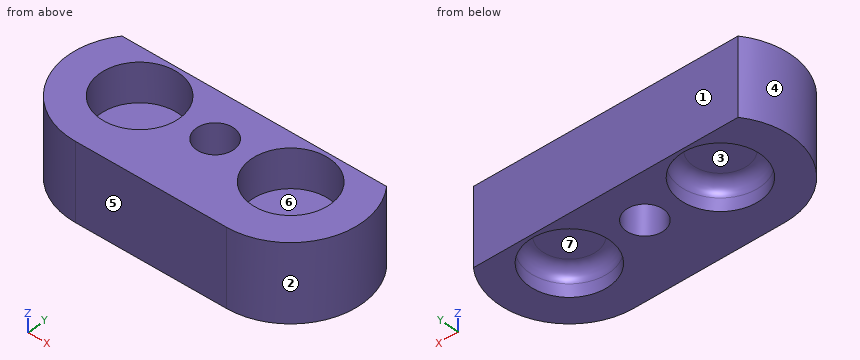
from build123d import *

# Parameters (mm, degrees)
SKETCH1_R           = 3.5
SKETCH1_R_2         = 3.1
EXTRUDE_THIN1_DEPTH = 2
BOSS_EXTRUDE1_DEPTH = 4
SKETCH3_R           = 3.05
CUT_EXTRUDE1_DEPTH  = 3
CUT_EXTRUDE2_REACH  = 15.016
SKETCH4_R           = 1.45
BOSS_EXTRUDE2_START = 2
SKETCH5_R           = 1.45
BOSS_EXTRUDE2_DEPTH = 2
FILLET1_R           = 1
EXTRUDE_THIN2_START = -6
EXTRUDE_THIN2_DEPTH = 6
CUT_EXTRUDE3_REACH  = 17.557


with BuildPart() as part:
    # Sketch1 → Extrude-Thin1 (new body)
    with BuildSketch(Plane.XY):
        with Locations((-5.8, 3.35)):
            Circle(SKETCH1_R)
        with Locations((-5.8, 3.35)):
            Circle(SKETCH1_R_2, mode=Mode.SUBTRACT)
    extrude(amount=EXTRUDE_THIN1_DEPTH)


with BuildPart() as body_2:
    # Mirror3: mirrored copy
    add(part.part.mirror(Plane(origin=(0, 0, 0), x_dir=(0, 0, 1), z_dir=(1, 0, 0))))


with BuildPart() as part_1:
    add(part.part)

    add(body_2.part)  # Boss-Extrude1 merges body 2
    # Sketch2 → Boss-Extrude1 (add)
    with BuildSketch(Plane.XY.offset(2)):
        with BuildLine():
            Line((-5.8, 6.85), (5.8, 6.85))
            ThreePointArc((5.8, 6.85), (9.3, 3.35), (5.8, -0.15))
            Line((5.8, -0.15), (-5.8, -0.15))
            ThreePointArc((-5.8, -0.15), (-9.3, 3.35), (-5.8, 6.85))
        make_face()
    extrude(amount=BOSS_EXTRUDE1_DEPTH)

    # Sketch3 → Cut-Extrude1 (cut)
    with BuildSketch(Plane.XY.offset(6)):
        with Locations((-5.8, 3.35)):
            Circle(SKETCH3_R)
    cut_extrude1 = extrude(amount=-CUT_EXTRUDE1_DEPTH, mode=Mode.SUBTRACT)

    # Mirror4: Cut-Extrude1 across plane
    add(cut_extrude1.mirror(Plane(origin=(0, 0, 0), x_dir=(0, 0, 1), z_dir=(1, 0, 0))), mode=Mode.SUBTRACT)

    # Sketch4 → Cut-Extrude2 (cut, up to next)
    with BuildSketch(Plane.XY.offset(6), mode=Mode.PRIVATE) as cut_extrude2_sk1:
        with Locations((0, 3.35)):
            Circle(SKETCH4_R)
    cut_extrude2_tool1 = extrude(cut_extrude2_sk1.sketch, amount=-CUT_EXTRUDE2_REACH, mode=Mode.PRIVATE) & part_1.part
    add(cut_extrude2_tool1.solids().sort_by_distance((0, 3.35, 6))[0], mode=Mode.SUBTRACT)

    # Sketch5 → Boss-Extrude2 (add)
    with BuildSketch(Plane(origin=(0, 0, 2), x_dir=(-1, 0, 0), z_dir=(0, 0, -1)).offset(BOSS_EXTRUDE2_START)):
        with BuildLine():
            Line((-5.8, -0.15), (5.8, -0.15))
            ThreePointArc((5.8, -0.15), (2.3, 3.35), (5.8, 6.85))
            Line((5.8, 6.85), (-5.8, 6.85))
            ThreePointArc((-5.8, 6.85), (-2.3, 3.35), (-5.8, -0.15))
        make_face()
        with Locations(Location((0, 3.35, 0), (0, 0, 180))):
            Circle(SKETCH5_R, mode=Mode.SUBTRACT)
    extrude(amount=-BOSS_EXTRUDE2_DEPTH)

    # Fillet1
    fillet1_edges = [part_1.edges().sort_by_distance(p)[0] for p in [
        (-8.9, 3.35, 2),
        (8.9, 3.35, 2),
    ]]
    fillet(fillet1_edges, radius=FILLET1_R)

    # Sketch6 → Extrude-Thin2 (add)
    with BuildSketch(Plane.XY.offset(6).offset(EXTRUDE_THIN2_START)):
        with BuildLine():
            Line((5.8, 8.85), (-5.8, 8.85))
            ThreePointArc((-5.8, 8.85), (-11.3, 3.35), (-5.8, -2.15))
            Line((-5.8, -2.15), (5.8, -2.15))
            ThreePointArc((5.8, -2.15), (11.3, 3.35), (5.8, 8.85))
        make_face()
        with BuildLine():
            Line((5.8, 6.85), (-5.8, 6.85))
            ThreePointArc((-5.8, 6.85), (-9.3, 3.35), (-5.8, -0.15))
            Line((-5.8, -0.15), (5.8, -0.15))
            ThreePointArc((5.8, -0.15), (9.3, 3.35), (5.8, 6.85))
        make_face(mode=Mode.SUBTRACT)
    extrude(amount=EXTRUDE_THIN2_DEPTH)

    # Sketch7 → Cut-Extrude3 (cut, up to next)
    with BuildSketch(Plane.XY.offset(6), mode=Mode.PRIVATE) as cut_extrude3_sk1:
        with BuildLine():
            Line((-10.162052269, 6.7), (10.162052269, 6.7))
            ThreePointArc((10.162052269, 6.7), (8.231563283, 8.28330518), (5.8, 8.85))
            Line((5.8, 8.85), (-5.8, 8.85))
            ThreePointArc((-5.8, 8.85), (-8.231563283, 8.28330518), (-10.162052269, 6.7))
        make_face()
    cut_extrude3_tool1 = extrude(cut_extrude3_sk1.sketch, amount=-CUT_EXTRUDE3_REACH, mode=Mode.PRIVATE) & part_1.part
    add(cut_extrude3_tool1.solids().sort_by_distance((0, 7.706585, 6))[0], mode=Mode.SUBTRACT)


solid = part_1.part
Geometry: final body of the model. Coordinates: model frame, mm. Face numbers are marked on the shaded views. A direction names the side the tool comes from. Round coordinates to 2 decimals unless told otherwise and drop trailing zeros. Order: outer loops, then holes, each group sorted by start corner. A loop starts at its lowest first (then second) coordinate and runs counter-clockwise, first axis right, second up. Notation, with made-up numbers: (-32, 49.25) -> (23, 49.25) arc R32 ccw to (23, 87.25) -> close; hole circle Ø9 at (-38.75, 76). An arc over 180 degrees is marked (long way). Put each result on its own line as item: value. Start each with the question number.
Q1. Section C-C on z = 4.75. Return the cut outline in (x, y).
Q2. Section A-A on y = 3.35. Return the cut outline in (x, z), and give its area (3 significant figures).
Q3. Reachability of the marked faces 5, 6 and 7 from +Z, -Z, +X, -X, +Y, -Y: full face, straight path, thin tool, end or side. Return the list, or none.
Q4. Section D-D on z = 0.5. Return the cut outline in (x, y), and give its area (3 significant figures).
Q5. First-contact query: pin 1 (2 mm diameter, centred on y = 2, z = 1, fed in from -X); pin 2 (5 mm diameter, centred on x = 7.5, y = 3.5, fed in from +Z); pin 3 (5 mm diameter, centred on x = -5.8, y = 3.35, fed in from +Z); pin 4 (4.5 mm diameter, centred on x = -5.5, y = 3.5, fed in from -Z). Flat tips, straight axial feed; report the tip coordinate or a pass-through.
Q6. Line query: probe 1 along X at (y, z) = (3.35, 2.7); probe 2 along Y at (x, z) = (5.8, 3.95); probe 3 along X at (y, z) = (5, 0.8). Output: solid intervals per line, ascending.
Q7. Pull-direction query (X, two-part tool) for the marked faces 1, 2, 3 and 4; classes: +X half, -X half, draft (parallel to the pull), parting line (faces both ways), or undercut.
Q8. Section B-B on x = 0. Return the cut outline in (y, z).
Ans:
1. outline: (-10.16, 6.7) arc R5.5 ccw to (-5.8, -2.15) -> (5.8, -2.15) arc R5.5 ccw to (10.16, 6.7) -> close; hole circle Ø6.1 at (-5.8, 3.35); hole circle Ø2.9 at (0, 3.35); hole circle Ø6.1 at (5.8, 3.35)
2. outline: (-11.3, 0) -> (-8.9, 0) -> (-8.9, 1) arc R1 cw to (-7.9, 2) -> (-3.7, 2) arc R1 cw to (-2.7, 1) -> (-2.7, 0) -> (-1.45, 0) -> (-1.45, 6) -> (-2.75, 6) -> (-2.75, 3) -> (-8.85, 3) -> (-8.85, 6) -> (-11.3, 6) -> close; (1.45, 0) -> (2.7, 0) -> (2.7, 1) arc R1 cw to (3.7, 2) -> (7.9, 2) arc R1 cw to (8.9, 1) -> (8.9, 0) -> (11.3, 0) -> (11.3, 6) -> (8.85, 6) -> (8.85, 3) -> (2.75, 3) -> (2.75, 6) -> (1.45, 6) -> close
2. area: 57.7 mm2
3. face 5: +Z, -Z, +X, -X, -Y
3. face 6: +Z
3. face 7: -Z
4. outline: (-10.16, 6.7) arc R5.5 ccw to (-5.8, -2.15) -> (5.8, -2.15) arc R5.5 ccw to (10.16, 6.7) -> close; hole circle Ø6.2 at (-5.8, 3.35); hole circle Ø2.9 at (0, 3.35); hole circle Ø6.2 at (5.8, 3.35)
4. area: 118 mm2
5. pin 1: stops at x = -11.29
5. pin 2: stops at z = 6
5. pin 3: stops at z = 3
5. pin 4: stops at z = 1.87
6. probe 1: x = -11.3 to -1.45, 1.45 to 11.3
6. probe 2: y = -2.15 to 0.3, 6.4 to 6.7
6. probe 3: x = -11.05 to -8.42, -3.18 to 3.18, 8.42 to 11.05
7. face 1: draft
7. face 2: +X half
7. face 3: undercut
7. face 4: -X half
8. outline: (-2.15, 0) -> (1.9, 0) -> (1.9, 6) -> (-2.15, 6) -> close; (4.8, 0) -> (6.7, 0) -> (6.7, 6) -> (4.8, 6) -> close
